from build123d import *

# Parameters (mm, degrees)
SKETCH_1_R      = 1.65
SKETCH_1_R_2    = 6.75
SKETCH_1_R_3    = 1.6
EXTRUDE_1_DEPTH = 3
FILLET_1_R      = 5


with BuildPart() as part:
    # ｽｹｯﾁ1 → ﾎﾞｽ - 押し出し1 (new body)
    with BuildSketch(Plane(origin=(0, 0, 0), x_dir=(1, 0, 0), z_dir=(0, 1, 0))):
        with BuildLine():
            Line((0, 0), (9.387505004, 0))
            ThreePointArc((9.387505004, 0), (25, 2.5), (40.612494996, 0))
            Line((40.612494996, 0), (50, 0))
            Line((50, 0), (50, 30))
            Line((50, 30), (0, 30))
            Line((0, 30), (0, 0))
        make_face()
        with Locations(Location((45, 5, 0), (0, 0, 270))):
            Circle(SKETCH_1_R, mode=Mode.SUBTRACT)
        with Locations(Location((5, 5, 0), (0, 0, 90))):
            Circle(SKETCH_1_R, mode=Mode.SUBTRACT)
        with Locations(Location((5, 25, 0), (0, 0, 270))):
            Circle(SKETCH_1_R, mode=Mode.SUBTRACT)
        with Locations(Location((45, 25, 0), (0, 0, 90))):
            Circle(SKETCH_1_R, mode=Mode.SUBTRACT)
        with Locations(Location((25, 15, 0), (0, 0, 270))):
            Circle(SKETCH_1_R_2, mode=Mode.SUBTRACT)
        with Locations(Location((25, 24.5, 0), (0, 0, 270))):
            Circle(SKETCH_1_R_3, mode=Mode.SUBTRACT)
        with Locations(Location((33.227241336, 10.25, 0), (0, 0, 270))):
            Circle(SKETCH_1_R_3, mode=Mode.SUBTRACT)
        with Locations(Location((16.772758664, 10.25, 0), (0, 0, 270))):
            Circle(SKETCH_1_R_3, mode=Mode.SUBTRACT)
    extrude(amount=EXTRUDE_1_DEPTH)

    # ﾌｨﾚｯﾄ1
    fillet_1_edges = [part.edges().sort_by_distance(p)[0] for p in [
        (0, 1.5, -30),
        (50, 1.5, -30),
        (50, 1.5, 0),
        (40.612494996, 1.5, 0),
        (9.387505004, 1.5, 0),
        (0, 1.5, 0),
    ]]
    fillet(fillet_1_edges, radius=FILLET_1_R)


solid = part.part
CAD build for the part. Positions are in the model's coordinates, mm. A direction names the side the tool comes from. Round coordinates to 2 decimals unless told otherwise and drop trailing zeros. Loops run counter-clockwise (first coordinate to the right, second up) from the corner with the lowest first, then second, coordinate; pieces in that order, holes last. Notation, with made-up numbers: (72, 87) - (104, 87) arc R20 cw to (104, 108) - close; hole circle Ø5 at (26.25, 10). An arc over 180 degrees is marked (long way). Put each result on its own line as item: value.
1. Two-plate mould, pull along X, no slides. Class faces 1 (the flat face through (25, 0, -22)), 2 (the cylindrical face through (24.8, 1.5, -2.5)), 3 (the flat face through (50, 1, -15)): released by +X, released by -X, zero draft, split by the parting line, or undercut.
Geometry check:
face 1: zero draft
face 2: undercut
face 3: released by +X
2. Wall check: line 1 (X direction, y = 2.1, z = -25); line 2 (X direction, y = 1.15, z = -24.5); line 3 (Z direction, x = 5.5, y = 0.65). Give the ranges that are in metal, low to high.
Geometry check:
line 1: 0 to 3.35, 6.65 to 23.48, 26.52 to 43.35, 46.65 to 50
line 2: 0 to 3.43, 6.57 to 23.4, 26.6 to 43.43, 46.57 to 50
line 3: -30 to -26.57, -23.43 to -6.57, -3.43 to 0
3. Pin check, flat tip, straight feed: P1, Ø3, axis at x = 16.77, z = -10.25, coming from the -Y side. Stop position of the tip, or through.
Geometry check:
P1: through
4. Slice it at D-D on y = 1.6. Give the number of separate pieces and of enclosed holes in the cut face, and give its area (3 significant figures).
Geometry check:
separate pieces: 1
enclosed holes: 8
area: 1,220 mm²
5. Slice it at A-A on z = -15. List the corners of the cut face in (x, y), and give its area (4 significant figures).
Geometry check:
outline: (0, 0) - (18.25, 0) - (18.25, 3) - (0, 3) - close; (31.75, 0) - (50, 0) - (50, 3) - (31.75, 3) - close
area: 109.5 mm²
6. Slice it at C-C on z = -24.25. List the corners of the cut face in (x, y), and give its area (3 significant figures).
Geometry check:
outline: (0, 0) - (3.53, 0) - (3.53, 3) - (0, 3) - close; (6.47, 0) - (23.42, 0) - (23.42, 3) - (6.47, 3) - close; (26.58, 0) - (43.53, 0) - (43.53, 3) - (26.58, 3) - close; (46.47, 0) - (50, 0) - (50, 3) - (46.47, 3) - close
area: 123 mm²
7. 3-axis set-ups, long thin cutter, end or side, ignore diameter. For faces 4 (the cylindrical face through (9.35, 1.521, -0.056)), 5 (the cylindrical face through (15.8, 1.48, -11.52)): which of +Z, -Z, +X, -X, +Y, -Y reach the whole face in a straight line?
Geometry check:
face 4: +Z, +Y, -Y
face 5: +Y, -Y
8. Slice it at B-B on x = 25. List the corners of the cut face in (y, z).
Geometry check:
outline: (0, -30) - (3, -30) - (3, -26.1) - (0, -26.1) - close; (0, -22.9) - (3, -22.9) - (3, -21.75) - (0, -21.75) - close; (0, -8.25) - (3, -8.25) - (3, -2.5) - (0, -2.5) - close
